Check sheet for the modelled part. Datum: model origin and axes. Units: mm. A direction names the side the tool comes from. Coordinates: 2 decimals unless noted, no trailing zeros. Loops run counter-clockwise (first coordinate to the right, second up) from the corner with the lowest first, then second, coordinate; pieces in that order, holes last. Notation, with made-up numbers: (17, -29) -> (55, -29) arc R29 cw to (55, -1) -> close; hole circle Ø11 at (4.5, -14.75). An arc over 180 degrees is marked (long way). Use CSV: the item, a comma, the result in double quotes. Start each with the question number.
1. Sectioned sample at A-A, the plane z = -4.25. Record the cut outline in (x, y).
2. Sectioned sample at C-C, the plane x = -1. Record the cut outline in (y, z).
3. Sectioned sample at B-B, the plane y = 1.25. Record the cut outline in (x, z), and give its area (3 significant figures).
4. Sectioned sample at D-D, the plane z = 7. Record the cut outline in (x, y), and give its area (3 significant figures).
5. Set-up check for faces 1 (the face through (0, 8, -7.9)), 2 (the face through (-6.9, 13, 4)): record each of +Z, -Z, +X, -X, +Y, -Y from which the full face is reachable in a straight line by a thin tool's end or side.
6. Gauge pin test, flat ends, axial feed: pin 1 (2 mm diameter, centred on y = 9, z = -1.5, fed in from +X); pin 2 (2 mm diameter, centred on x = 0, y = 8, fed in from +Z); pin 3 (7 mm diameter, centred on x = -1, z = 1, fed in from +Y). Record the tip position at first contact, or that the pin passes through.
7. Thickness scan on L1, parallel to X at y = 11.5, z = 0.25; L2, parallel to Y at x = 2.5, z = -2; L3, parallel to X at y = 14.75, z = -1.75. Record the ranges inside material, lowest first.
```python
from build123d import *

# Parameters (mm, degrees)
ESQUISSE1_W                  = 15.8
ESQUISSE1_H                  = 15.8
BOSS_EXTRU_1_DEPTH           = 15.8
COQUE1_T                     = -2
ENL_V_MAT_EXTRU_1_DEPTH      = 3.5
ENL_V_MAT_EXTRU_2_DEPTH      = 3.5
ENL_V_MAT_EXTRU_3_DEPTH      = 24.7
ENL_V_MAT_EXTRU_3_DEPTH_BACK = 3.5
CONG_1_R                     = 1
CHANFREIN1_SIZE              = 0.4


with BuildPart() as part:
    # Esquisse1 → Boss.-Extru.1 (new body)
    with BuildSketch(Plane(origin=(0, 0, 0), x_dir=(1, 0, 0), z_dir=(0, 1, 0))):
        Rectangle(ESQUISSE1_W, ESQUISSE1_H)
    extrude(amount=BOSS_EXTRU_1_DEPTH)

    # Coque1
    coque1_openings = [part.faces().sort_by_distance(p)[0] for p in [
        (0, 15.8, 0),
        (0, 7.9, 7.9),
        (7.9, 7.9, 0),
    ]]
    offset(amount=COQUE1_T, openings=coque1_openings, kind=Kind.INTERSECTION)

    # Esquisse2 → Enlèv. mat.-Extru.1 (cut)
    with BuildSketch(Plane.XY.offset(7.9)):
        Polygon((-5.9, 15.8), (-6.9, 15.8), (-6.9, 1), (7.9, 1), (7.9, 2), (-5.9, 2), align=None)
    extrude(amount=-ENL_V_MAT_EXTRU_1_DEPTH, mode=Mode.SUBTRACT)

    # Esquisse6 → Enlèv. mat.-Extru.2 (cut)
    with BuildSketch(Plane(origin=(0, 15.8, 0), x_dir=(1, 0, 0), z_dir=(0, 1, 0))):
        Polygon((-5.9, -4.4), (-5.9, 5.9), (7.9, 5.9), (7.9, 6.9), (-6.9, 6.9), (-6.9, -4.4), align=None)
    extrude(amount=-ENL_V_MAT_EXTRU_2_DEPTH, mode=Mode.SUBTRACT)

    # Esquisse7 → Enlèv. mat.-Extru.3 (cut, two sides: drawn at the far end of the back side and taken through both)
    with BuildSketch(Plane(origin=(7.9, 0, 0), x_dir=(0, 0, -1), z_dir=(1, 0, 0)).offset(-ENL_V_MAT_EXTRU_3_DEPTH_BACK)):
        Polygon((5.9, 2), (-4.4, 2), (-4.4, 1), (6.9, 1), (6.9, 12.3), (5.9, 12.3), align=None)
    extrude(amount=ENL_V_MAT_EXTRU_3_DEPTH + ENL_V_MAT_EXTRU_3_DEPTH_BACK, mode=Mode.SUBTRACT)

    # Congé1
    cong_1_edges = [part.edges().sort_by_distance(p)[0] for p in [
        (-5.9, 2, -0.75),
        (-5.9, 7.15, -5.9),
        (-0.75, 2, -5.9),
    ]]
    fillet(cong_1_edges, radius=CONG_1_R)

    # Chanfrein1
    chanfrein1_edges = [part.edges().sort_by_distance(p)[0] for p in [
        (-5.9, 7.65, 4.4),
        (-6.4, 12.3, 4.4),
        (-5.9, 12.3, -0.25),
        (-0.25, 2, 4.4),
        (4.4, 2, -0.25),
        (4.4, 12.3, -6.4),
        (4.4, 1.5, 4.4),
        (4.4, 7.65, -5.9),
        (-0.25, 12.3, -5.9),
        (-5.607106781, 12.3, -5.607106781),
        (4.4, 2.292893219, -5.607106781),
        (-5.607106781, 2.292893219, 4.4),
    ]]
    chamfer(chanfrein1_edges, length=CHANFREIN1_SIZE)


solid = part.part
```
Completed:
1,outline,"(-7.9, 0) -> (7.9, 0) -> (7.9, 1) -> (4.4, 1) -> (4.4, 1.6) -> (4, 2) -> (-4.9, 2) arc R1 cw to (-5.9, 3) -> (-5.9, 11.9) -> (-6.3, 12.3) -> (-6.9, 12.3) -> (-6.9, 15.8) -> (-7.9, 15.8) -> close"
2,outline,"(0, -7.9) -> (15.8, -7.9) -> (15.8, -6.9) -> (12.3, -6.9) -> (12.3, -6.3) -> (11.9, -5.9) -> (3, -5.9) arc R1 cw to (2, -4.9) -> (2, 4) -> (1.6, 4.4) -> (1, 4.4) -> (1, 7.9) -> (0, 7.9) -> close"
3,outline,"(-7.9, -7.9) -> (7.9, -7.9) -> (7.9, -6.9) -> (4.4, -6.9) -> (4.4, 4) -> (4, 4.4) -> (-6.9, 4.4) -> (-6.9, 7.9) -> (-7.9, 7.9) -> close"
3,area,"158 mm²"
4,outline,"(-7.9, 0) -> (7.9, 0) -> (7.9, 1) -> (-6.9, 1) -> (-6.9, 15.8) -> (-7.9, 15.8) -> close"
4,area,"30.6 mm²"
5,face 1,"-Z, +X, -X, +Y, -Y"
5,face 2,"+Z, +X, +Y"
6,pin 1,"x = -5.9"
6,pin 2,"z = -5.9"
6,pin 3,"y = 2"
7,L1,"-7.9 to -5.9"
7,L2,"0 to 2"
7,L3,"-7.9 to -6.9"
